Check sheet for the modelled part. Datum: model origin and axes. Units: mm. A direction names the side the tool comes from. Round coordinates to 2 decimals unless told otherwise and drop trailing zeros. Write each loop counter-clockwise with the first axis right and the second up, starting at its lowest first coordinate (ties: lowest second). Pieces come first, ordered by that corner, then holes. Notation, with made-up numbers: M -11,50.5 L 41,50.5 A29 cw 41,76.5 Z; hole C -24,-33.75 d6. An arc over 180 degrees is marked long. Answer in a Markdown table with one row per item.
```python
from build123d import *

# Parameters (mm, degrees)
BOSS_EXTRUDE1_DEPTH = 6.35
SKETCH20_R          = 35
BOSS_EXTRUDE5_DEPTH = 19.05
CUT_EXTRUDE14_DEPTH = 128.996314535
CHAMFER1_SIZE       = 19.05
SKETCH22_R          = 3.175
CUT_EXTRUDE15_DEPTH = 135.156064825
SKETCH24_R          = 5
CUT_EXTRUDE16_DEPTH = 140.018309755
SKETCH25_R          = 2.38125
CUT_EXTRUDE17_DEPTH = 10
CUT_EXTRUDE18_DEPTH = 10


with BuildPart() as part:
    # Sketch1 → Boss-Extrude1 (new body)
    with BuildSketch(Plane(origin=(0, 0, 0), x_dir=(0, 0, -1), z_dir=(1, 0, 0))):
        with BuildLine():
            Line((-34.968464441, 1.48542743), (-25.35, -97.464164516))
            ThreePointArc((-25.35, -97.464164516), (0, -120.469483831), (25.35, -97.464164516))
            Line((25.35, -97.464164516), (34.968464441, 1.48542743))
            ThreePointArc((34.968464441, 1.48542743), (0, 35), (-34.968464441, 1.48542743))
        make_face()
        Polygon((4.353205728, 11.960334439), (-11.960334439, 4.353205728), (-4.353205728, -11.960334439), (11.960334439, -4.353205728), align=None, mode=Mode.SUBTRACT)
    extrude(amount=BOSS_EXTRUDE1_DEPTH)

    # Sketch20 → Boss-Extrude5 (add)
    with BuildSketch(Plane(origin=(6.35, 0, 0), x_dir=(0, 0, -1), z_dir=(1, 0, 0))):
        with Locations(Location((0, 0, 0), (0, 0, 177.567591624))):
            Circle(SKETCH20_R)
    extrude(amount=BOSS_EXTRUDE5_DEPTH)

    # Sketch21 → Cut-Extrude14 (cut, through all)
    with BuildSketch(Plane.ZY):
        Polygon((-19.067760927, 15.897892729), (-24.435012851, 4.387783834), (-10.840396045, -1.951490092), (-5.473144121, 9.558618803), align=None)
        Polygon((-11.960334439, -4.353205728), (-4.353205728, 11.960334439), (11.960334439, 4.353205728), (4.353205728, -11.960334439), align=None)
        Polygon((10.840396045, 1.951490092), (5.473144121, -9.558618803), (19.067760927, -15.897892729), (24.435012851, -4.387783834), align=None)
    extrude(amount=-CUT_EXTRUDE14_DEPTH, mode=Mode.SUBTRACT)

    # Chamfer1
    # the kernel refuses this chamfer: 19.05 mm, written as the material it takes off along each edge
    with BuildSketch(Plane(origin=(25.4, 0, 0), x_dir=(0, 0.042440783710504346, 0.9990989840241247), z_dir=(0, 0.9990989840241247, -0.042440783710504346))) as chamfer1_piece_1:
        Polygon((35, -CHAMFER1_SIZE), (35 - CHAMFER1_SIZE, 0), (35, 0), align=None)
    revolve(axis=Axis((25.4, 0, 0), (1, 0, 0)), mode=Mode.SUBTRACT)

    # Sketch22 → Cut-Extrude15 (cut, through all)
    with BuildSketch(Plane(origin=(0, 5.755054448, 2.683625962), x_dir=(-1, 0, 0), z_dir=(0, -0.9063077870366495, -0.4226182617407006))):
        with Locations(Location((-13.4, -16.5, 0), (0, 0, 90))):
            Circle(SKETCH22_R)
    cut_extrude15 = extrude(amount=-CUT_EXTRUDE15_DEPTH, mode=Mode.SUBTRACT)

    # Sketch24 → Cut-Extrude16 (cut, through all)
    with BuildSketch(Plane(origin=(0, 10.286593383, 4.796717271), x_dir=(-1, 0, 0), z_dir=(0, -0.9063077870366495, -0.4226182617407006))):
        with Locations(Location((-13.4, -16.5, 0), (0, 0, 90))):
            Circle(SKETCH24_R)
    cut_extrude16 = extrude(amount=-CUT_EXTRUDE16_DEPTH, mode=Mode.SUBTRACT)

    # Sketch25 → Cut-Extrude17 (cut)
    with BuildSketch(Plane(origin=(0, -5.755054448, -2.683625962), x_dir=(1, 0, 0), z_dir=(0, 0.9063077870366495, 0.4226182617407006))):
        with Locations(Location((13.4, -16.5, 0), (0, 0, 270))):
            Circle(SKETCH25_R)
    cut_extrude17 = extrude(amount=-CUT_EXTRUDE17_DEPTH, mode=Mode.SUBTRACT)

    # Mirror1: Cut-Extrude15, Cut-Extrude16, Cut-Extrude17 across plane
    add(cut_extrude15.mirror(Plane(origin=(0, 0, 0), x_dir=(1, 0, 0), z_dir=(0, 0.42261826174070105, -0.9063077870366493))), mode=Mode.SUBTRACT)
    add(cut_extrude16.mirror(Plane(origin=(0, 0, 0), x_dir=(1, 0, 0), z_dir=(0, 0.42261826174070105, -0.9063077870366493))), mode=Mode.SUBTRACT)
    add(cut_extrude17.mirror(Plane(origin=(0, 0, 0), x_dir=(1, 0, 0), z_dir=(0, 0.42261826174070105, -0.9063077870366493))), mode=Mode.SUBTRACT)

    # Sketch19 → Cut-Extrude18 (cut)
    with BuildSketch(Plane(origin=(6.35, 0, 0), x_dir=(0, 0, -1), z_dir=(1, 0, 0))):
        with BuildLine():
            Line((13.556349186, -69.583650814), (13.556349186, -79.583650814))
            ThreePointArc((13.556349186, -79.583650814), (15.556349186, -81.583650814), (17.556349186, -79.583650814))
            Line((17.556349186, -79.583650814), (17.556349186, -69.583650814))
            ThreePointArc((17.556349186, -69.583650814), (15.556349186, -67.583650814), (13.556349186, -69.583650814))
        make_face()
        with BuildLine():
            Line((-10, -85.14), (-10, -95.14))
            ThreePointArc((-10, -95.14), (0, -105.14), (10, -95.14))
            Line((10, -95.14), (10, -85.14))
            ThreePointArc((10, -85.14), (0, -75.14), (-10, -85.14))
        make_face()
        with BuildLine():
            Line((17.556349186, -110.696349186), (17.556349186, -100.696349186))
            ThreePointArc((17.556349186, -100.696349186), (15.556349186, -98.696349186), (13.556349186, -100.696349186))
            Line((13.556349186, -100.696349186), (13.556349186, -110.696349186))
            ThreePointArc((13.556349186, -110.696349186), (15.556349186, -112.696349186), (17.556349186, -110.696349186))
        make_face()
        with BuildLine():
            Line((-17.556349186, -69.583650814), (-17.556349186, -79.583650814))
            ThreePointArc((-17.556349186, -79.583650814), (-15.556349186, -81.583650814), (-13.556349186, -79.583650814))
            Line((-13.556349186, -79.583650814), (-13.556349186, -69.583650814))
            ThreePointArc((-13.556349186, -69.583650814), (-15.556349186, -67.583650814), (-17.556349186, -69.583650814))
        make_face()
        with BuildLine():
            Line((-13.556349186, -110.696349186), (-13.556349186, -100.696349186))
            ThreePointArc((-13.556349186, -100.696349186), (-15.556349186, -98.696349186), (-17.556349186, -100.696349186))
            Line((-17.556349186, -100.696349186), (-17.556349186, -110.696349186))
            ThreePointArc((-17.556349186, -110.696349186), (-15.556349186, -112.696349186), (-13.556349186, -110.696349186))
        make_face()
    extrude(amount=-CUT_EXTRUDE18_DEPTH, mode=Mode.SUBTRACT)


with BuildPart() as body_2:
    # Mirror2: mirrored copy
    add(part.part.mirror(Plane(origin=(0, 0, 0), x_dir=(0, 0, 1), z_dir=(1, 0, 0))))


solid = body_2.part
```
1. Section check A-A, the plane x = -20.5. Record the cut outline in (y, z).
Found:
| item | result |
|---|---|
| outline | M -14.15,15.32 A20.85 ccw 2.64,-20.68 L -1.95,-10.84 L -4.35,-11.96 L -11.96,4.35 L -9.56,5.47 Z; M -2.64,20.68 L 1.95,10.84 L 4.35,11.96 L 11.96,-4.35 L 9.56,-5.47 L 14.15,-15.32 A20.85 ccw Z |
2. Access from +Z, -Z, +X, -X, +Y, -Y to the whole of each face (thin tool, end or side, straight path). Record for faces 4 (the face through (-3.219, -98.697, -15.6)), 5 (the face through (-10.14, 3.75, 18.81)).
Found:
| item | result |
|---|---|
| face 4 | +X, -X |
| face 5 | none |
3. Section check D-D, the plane y = -41. Record the cut outline in (x, z).
Found:
| item | result |
|---|---|
| outline | M -6.35,-30.84 L 0,-30.84 L 0,30.84 L -6.35,30.84 Z |
4. Draft check along Z on faces 1 (the face through (-24.48, -11.92, -11.94)), 2 (the face through (-3.131, -48.682, -30.092)), 3 (the face through (-3, -75, 13.556)). Enter one of: +Z half, -Z half, draft (parallel to the pull), parting line (faces both ways), or undercut.
Found:
| item | result |
|---|---|
| face 1 | parting line |
| face 2 | -Z half |
| face 3 | undercut |
5. Section check B-B, the plane x = -3.25. Count the separate pieces of the cut face and the enclosed holes in it, and give its area (3 significant figures).
Found:
| item | result |
|---|---|
| separate pieces | 1 |
| enclosed holes | 6 |
| area | 7,250 mm2 |
6. Scan lines: L1, parallel to Y at x = -12.75, z = -22; L2, parallel to Y at x = -21, z = -13.5; L3, parallel to Z at x = -3.5, y = -99.5. Record each from-to range of solid material in increasing order.
Found:
| item | result |
|---|---|
| L1 | y = -18.27 to -7.78, -2.72 to 3.25, 9.61 to 18.27 |
| L2 | y = -15.23 to -0.71, 13.3 to 15.23 |
| L3 | z = -25.07 to -17.16, -13.95 to -9, 9 to 13.95, 17.16 to 25.07 |
7. Go/stop test with flat-tipped pins: pin 1 (7 mm diameter, centred on x = -3.5, y = -73, fed in from +Z); pin 2 (2 mm diameter, centred on y = -92.5, z = 13, fed in from -X); pin 3 (12 mm diameter, centred on x = -17, y = -4.5, fed in from +Z). Record where each tip stops, or that it passes through.
Found:
| item | result |
|---|---|
| pin 1 | stops at z = 28.07 |
| pin 2 | stops at x = -6.35 |
| pin 3 | stops at z = 30.07 |
